```python
from build123d import *

# Parameters (mm, degrees)
SKETCH_1_W                         = 50
SKETCH_1_H                         = 95
SM_BASE_FLANGE_1_DEPTH             = 3
SM_EDGE_FLANGE_1_STRIP_W           = 13.4732
SM_EDGE_FLANGE_1_STRIP_H           = 3
SM_EDGE_FLANGE_1_STRIP_CUT_DEPTH   = 50
SM_EDGE_FLANGE_1_STRIP_2_W         = 13.4732
SM_EDGE_FLANGE_1_STRIP_2_H         = 3
SM_EDGE_FLANGE_1_STRIP_CUT_2_DEPTH = 50
SM_EDGE_FLANGE_1_DEPTH             = 50
SM_EDGE_FLANGE_1_BEND_DEPTH        = 50
SM_EDGE_FLANGE_2_STRIP_W           = 13.4732
SM_EDGE_FLANGE_2_STRIP_H           = 3
SM_EDGE_FLANGE_2_STRIP_CUT_DEPTH   = 50
SM_EDGE_FLANGE_2_STRIP_2_W         = 13.4732
SM_EDGE_FLANGE_2_STRIP_2_H         = 3
SM_EDGE_FLANGE_2_STRIP_CUT_2_DEPTH = 50
SM_EDGE_FLANGE_2_DEPTH             = 50
SM_EDGE_FLANGE_2_BEND_DEPTH        = 50
SKETCH_18_R                        = 6.5
CUT_EXTRUDE_1_DEPTH                = 137.579647093


# Sheet-metal steps are written as plain solids
with BuildPart() as part:
    # Sketch 1 → 基体-法兰1 (new body)
    with BuildSketch(Plane.XY):
        with Locations((25, 47.5)):
            Rectangle(SKETCH_1_W, SKETCH_1_H)
    extrude(amount=-SM_BASE_FLANGE_1_DEPTH)

    # 边线-法兰1 strip (across the edge) → 边线-法兰1 strip cut (cut)
    with BuildSketch(Plane(origin=(0, 95, -3), x_dir=(0, -1, 0), z_dir=(1, 0, 0))):
        with Locations((-6, -1.5)):
            Rectangle(SM_EDGE_FLANGE_1_STRIP_W, SM_EDGE_FLANGE_1_STRIP_H)
    extrude(amount=SM_EDGE_FLANGE_1_STRIP_CUT_DEPTH, mode=Mode.SUBTRACT)

    # 边线-法兰1 strip 2 (across the edge) → 边线-法兰1 strip cut 2 (cut)
    with BuildSketch(Plane(origin=(50, 0, -3), x_dir=(0, 1, 0), z_dir=(-1, 0, 0))):
        with Locations((-6, -1.5)):
            Rectangle(SM_EDGE_FLANGE_1_STRIP_2_W, SM_EDGE_FLANGE_1_STRIP_2_H)
    extrude(amount=SM_EDGE_FLANGE_1_STRIP_CUT_2_DEPTH, mode=Mode.SUBTRACT)

    # 边线-法兰1 section (across the edge) → 边线-法兰1 (add)
    with BuildSketch(Plane(origin=(0, 95, -3), x_dir=(0, -1, 0), z_dir=(1, 0, 0))):
        with BuildLine():
            Line((-3, 0.7366), (-3, 17))
            Line((-3, 17), (0, 17))
            Line((0, 17), (0, 0.7366))
            ThreePointArc((0, 0.7366), (0.215745145, 0.215745145), (0.7366, 0))
            Line((0.7366, 0), (0.7366, -3))
            ThreePointArc((0.7366, -3), (-1.905575199, -1.905575199), (-3, 0.7366))
        make_face()
    extrude(amount=SM_EDGE_FLANGE_1_DEPTH)

    # 边线-法兰1 section 2 (across the edge) → 边线-法兰1 bend (add)
    with BuildSketch(Plane(origin=(50, 0, -3), x_dir=(0, 1, 0), z_dir=(-1, 0, 0))):
        with BuildLine():
            Line((-3, 0.7366), (-3, 17))
            Line((-3, 17), (0, 17))
            Line((0, 17), (0, 0.7366))
            ThreePointArc((0, 0.7366), (0.215745145, 0.215745145), (0.7366, 0))
            Line((0.7366, 0), (0.7366, -3))
            ThreePointArc((0.7366, -3), (-1.905575199, -1.905575199), (-3, 0.7366))
        make_face()
    extrude(amount=SM_EDGE_FLANGE_1_BEND_DEPTH)

    # 边线-法兰2 strip (across the edge) → 边线-法兰2 strip cut (cut)
    with BuildSketch(Plane(origin=(0, -3, -20), x_dir=(0, 0, 1), z_dir=(1, 0, 0))):
        with Locations((-6, -1.5)):
            Rectangle(SM_EDGE_FLANGE_2_STRIP_W, SM_EDGE_FLANGE_2_STRIP_H)
    extrude(amount=SM_EDGE_FLANGE_2_STRIP_CUT_DEPTH, mode=Mode.SUBTRACT)

    # 边线-法兰2 strip 2 (across the edge) → 边线-法兰2 strip cut 2 (cut)
    with BuildSketch(Plane(origin=(50, 98, -20), x_dir=(0, 0, 1), z_dir=(-1, 0, 0))):
        with Locations((-6, -1.5)):
            Rectangle(SM_EDGE_FLANGE_2_STRIP_2_W, SM_EDGE_FLANGE_2_STRIP_2_H)
    extrude(amount=SM_EDGE_FLANGE_2_STRIP_CUT_2_DEPTH, mode=Mode.SUBTRACT)

    # 边线-法兰2 section (across the edge) → 边线-法兰2 (add)
    with BuildSketch(Plane(origin=(0, -3, -20), x_dir=(0, 0, 1), z_dir=(1, 0, 0))):
        with BuildLine():
            Line((-3, 0.7366), (-3, 27))
            Line((-3, 27), (0, 27))
            Line((0, 27), (0, 0.7366))
            ThreePointArc((0, 0.7366), (0.215745145, 0.215745145), (0.7366, 0))
            Line((0.7366, 0), (0.7366, -3))
            ThreePointArc((0.7366, -3), (-1.905575199, -1.905575199), (-3, 0.7366))
        make_face()
    extrude(amount=SM_EDGE_FLANGE_2_DEPTH)

    # 边线-法兰2 section 2 (across the edge) → 边线-法兰2 bend (add)
    with BuildSketch(Plane(origin=(50, 98, -20), x_dir=(0, 0, 1), z_dir=(-1, 0, 0))):
        with BuildLine():
            Line((-3, 0.7366), (-3, 27))
            Line((-3, 27), (0, 27))
            Line((0, 27), (0, 0.7366))
            ThreePointArc((0, 0.7366), (0.215745145, 0.215745145), (0.7366, 0))
            Line((0.7366, 0), (0.7366, -3))
            ThreePointArc((0.7366, -3), (-1.905575199, -1.905575199), (-3, 0.7366))
        make_face()
    extrude(amount=SM_EDGE_FLANGE_2_BEND_DEPTH)

    # 草图18 → 切除-拉伸1 (cut, through all)
    with BuildSketch(Plane.XY):
        with Locations((25, 47.5)):
            Circle(SKETCH_18_R)
    extrude(amount=-CUT_EXTRUDE_1_DEPTH, mode=Mode.SUBTRACT)


solid = part.part
```
Geometry: final body of the model. Coordinates: model frame, mm. A direction names the side the tool comes from. Give positions to 0.01 mm unless a question says otherwise; leave off trailing zeros. Loops run counter-clockwise (first coordinate to the right, second up) from the corner with the lowest first, then second, coordinate; pieces in that order, holes last. Notation, with made-up numbers: (-30.5, -14) -> (18.5, -14) arc R16 ccw to (18.5, 11) -> close; hole circle Ø7 at (44, 46.25). An arc over 180 degrees is marked (long way). Use CSV: the item, a comma, the result in double quotes.
(1) Cut plane D-D (x = 43.5). Output: boundary loops of the cut face in (y, z).
From the geometry:
outline,"(-30, -23) -> (-3.74, -23) arc R3.74 ccw to (0, -19.26) -> (0, -3.74) arc R0.74 cw to (0.74, -3) -> (94.26, -3) arc R0.74 cw to (95, -3.74) -> (95, -19.26) arc R3.74 ccw to (98.74, -23) -> (125, -23) -> (125, -20) -> (98.74, -20) arc R0.74 cw to (98, -19.26) -> (98, -3.74) arc R3.74 ccw to (94.26, 0) -> (0.74, 0) arc R3.74 ccw to (-3, -3.74) -> (-3, -19.26) arc R0.74 cw to (-3.74, -20) -> (-30, -20) -> close"
(2) Ray query, line 1 along Y through (x, z) = (12, -5.75); line 2 along Z through (x, y) = (13.5, 87); line 3 along Z through (x, y) = (28.5, 119.5). Return the intervals inside material, ascending. Write a range as [from, to].
From the geometry:
line 1,"[-3, 0], [95, 98]"
line 2,"[-3, 0]"
line 3,"[-23, -20]"
(3) Cut plane C-C (z = -9). Output: boundary loops of the cut face in (x, y).
From the geometry:
outline,"(0, -3) -> (50, -3) -> (50, 0) -> (0, 0) -> close; (0, 95) -> (50, 95) -> (50, 98) -> (0, 98) -> close"
(4) Pull-direction query (Y, two-part tool) for faces 6 (the face through (25, 59, -3)), 7 (the face through (25.35, -1.88, -1.07)), 8 (the face through (25, 125, -22)); classes: released by +Y, released by -Y, zero draft, split by the parting line, or undercut.
From the geometry:
face 6,"undercut"
face 7,"released by -Y"
face 8,"released by +Y"
(5) First-contact query: P1, Ø8, axis at x = 22.5, z = -9, coming from the -Y side; P2, Ø21, axis at x = 23, y = -12.5, coming from the +Z side; P3, Ø15, axis at x = 13.5, y = 57, coming from the -Z side; P4, Ø11.5, axis at x = 25, y = 47.5, coming from the +Z side. Flat tips, straight axial feed; report the tip coordinate or a pass-through.
From the geometry:
P1,"y = -3"
P2,"z = -1.19"
P3,"z = -3"
P4,"through"
(6) Access query for faces 1 (the face through (25, -17, -20)), 2 (the face through (0, 48, -2)), 3 (the face through (25, 112, -23)), 4 (the face through (24.65, -1.07, -21.88)), 5 (the face through (25, 112, -20)). Directions: +Z, -Z, +X, -X, +Y, -Y. A direction counts if a zero-diameter tool reaches every point of the face in a straight line with its end or side. Return the directions, or none.
From the geometry:
face 1,"+Z, +X, -X, -Y"
face 2,"+Z, -Z, -X, +Y, -Y"
face 3,"-Z, +X, -X, +Y, -Y"
face 4,"-Z, +X, -X"
face 5,"+Z, +X, -X, +Y"
(7) Cut plane A-A (y = 47.5). Output: boundary loops of the cut face in (x, z).
From the geometry:
outline,"(0, -3) -> (18.5, -3) -> (18.5, 0) -> (0, 0) -> close; (31.5, -3) -> (50, -3) -> (50, 0) -> (31.5, 0) -> close"
(8) Cut plane B-B (x = 25). Output: boundary loops of the cut face in (y, z).
From the geometry:
outline,"(-30, -23) -> (-3.74, -23) arc R3.74 ccw to (0, -19.26) -> (0, -3.74) arc R0.74 cw to (0.74, -3) -> (41, -3) -> (41, 0) -> (0.74, 0) arc R3.74 ccw to (-3, -3.74) -> (-3, -19.26) arc R0.74 cw to (-3.74, -20) -> (-30, -20) -> close; (54, -3) -> (94.26, -3) arc R0.74 cw to (95, -3.74) -> (95, -19.26) arc R3.74 ccw to (98.74, -23) -> (125, -23) -> (125, -20) -> (98.74, -20) arc R0.74 cw to (98, -19.26) -> (98, -3.74) arc R3.74 ccw to (94.26, 0) -> (54, 0) -> close"
